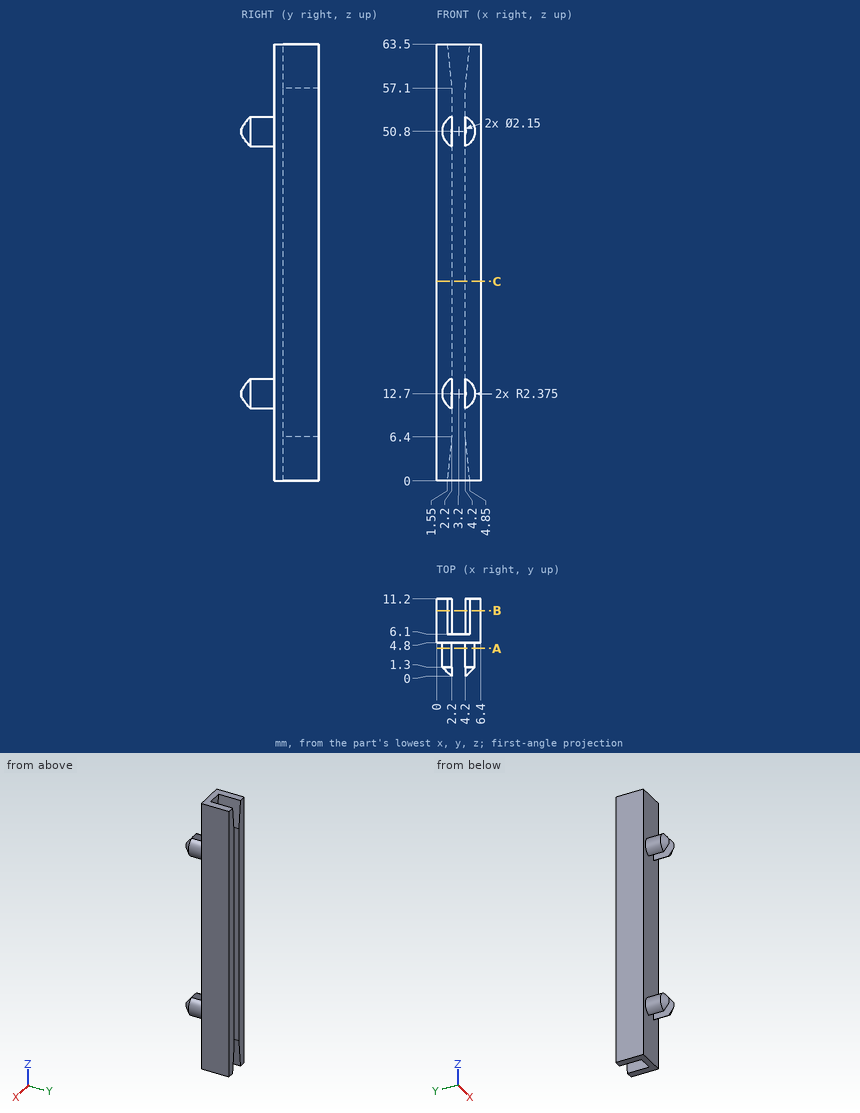
Print and shaded views of the part. All mm, measured from the part's lowest x, y and z. Coordinates: 2 decimals unless noted, no trailing zeros. Order: outer loops, then holes, each group sorted by start corner. A loop starts at its lowest first (then second) coordinate and runs counter-clockwise, first axis right, second up. Notation, with made-up numbers: M 89.25,-40 L 120.25,-40 A12 cw 120.25,-32 Z; hole C -39.75,43 d9. An arc over 180 degrees is marked long. Write each question's results on one line, items separated by ' | '. Start each with the question number.
Q1. Cut at A-A (y = 4). List the corners of the cut face in (x, z) (3 decimals), then the cut area to 3 significant figures.
Q2. Cut at B-B (y = 9.5). List the corners of the cut face in (x, z).
Q3. Cut at C-C (z = 29). List the corners of the cut face in (x, y), then the cut area to 3 significant figures.
Q4. Flat gauge pins, fed straight in: P1, Ø4.5, axis at y = 2.5, z = 51, coming from the +X side (3 decimals); P2, Ø2, axis at x = 5.5, z = 22.5, coming from the -Y side; P3, Ø2, axis at y = 2, z = 50.5, coming from the -X side (3 decimals). Where does each tip first touch, or does it go through?
Q5. Drill centre lines: probe 1 along X at (y, z) = (9.5, 54); probe 2 along Y at (x, z) = (3.25, 16); probe 3 along Y at (x, z) = (1.5, 34.5). Where is each one in solid material? Low to high. Write a range as from..to.
Found:
1) outline: M 2.2,10.546 L 2.2,14.854 A2.375 ccw Z; M 2.2,48.646 L 2.2,52.954 A2.375 ccw Z; M 4.2,10.546 A2.375 ccw 4.2,14.854 Z; M 4.2,48.646 A2.375 ccw 4.2,52.954 Z | area: 17.0 mm²
2) outline: M 0,0 L 1.55,0 L 2.2,6.4 L 2.2,57.1 L 1.55,63.5 L 0,63.5 Z; M 4.2,6.4 L 4.85,0 L 6.4,0 L 6.4,63.5 L 4.85,63.5 L 4.2,57.1 Z
3) outline: M 0,4.8 L 6.4,4.8 L 6.4,11.2 L 4.2,11.2 L 4.2,6.1 L 2.2,6.1 L 2.2,11.2 L 0,11.2 Z | area: 30.8 mm²
4) P1: x = 5.575 | P2: y = 4.8 | P3: x = 0.825
5) probe 1: 0..2.2, 4.2..6.4 | probe 2: 4.8..6.1 | probe 3: 4.8..11.2
